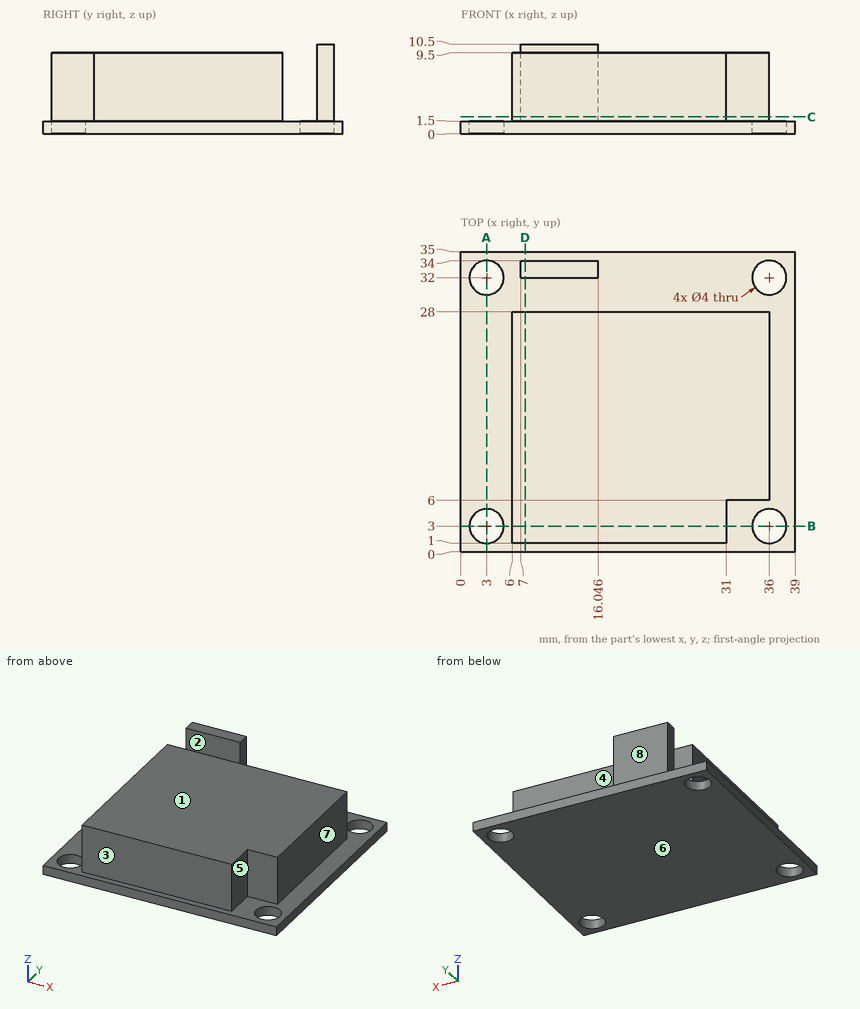
For this review, use the dimensioned drawing (mm, ordinates from the lowest corner) and the shaded views. A direction names the side the tool comes from. Coordinates: 2 decimals unless noted, no trailing zeros. Write each loop counter-clockwise with the first axis right and the second up, starting at its lowest first coordinate (ties: lowest second). Pieces come first, ordered by that corner, then holes. Notation, with made-up numbers: (-15, -19) - (33, -19) arc R15 ccw to (33, 5) - close; hole circle Ø4 at (-23.5, 36.5). An arc over 180 degrees is marked (long way). One line per item, written item: value.
1) Add section D-D (x = 7.5). State the section outline as (y, z) points, plus the area to 4 significant figures.
Answer sheet:
outline: (0, 0) - (35, 0) - (35, 1.5) - (34, 1.5) - (34, 10.5) - (32, 10.5) - (32, 1.5) - (28, 1.5) - (28, 9.5) - (1, 9.5) - (1, 1.5) - (0, 1.5) - close
area: 286.5 mm2
2) For the marked faces 5, 6, 7 and 8, list the 3-axis set-ups (+Z, -Z, +X, -X, +Y, -Y) from which the entire face can be reached by the end or side of a thin tool; tool diameter is ignored.
Answer sheet:
face 5: +Z, +X, -Y
face 6: -Z, +X, -X, +Y, -Y
face 7: +Z, +X, +Y, -Y
face 8: +Z, +X, -X, +Y
3) Insertion check: pin 1 (2 mm diameter, centred on x = 21.5, z = 6.5, fed in from +Y); pin 2 (2.5 mm diameter, centred on x = 13.5, z = 6.5, fed in from +Y); pin 3 (17.5 mm diameter, centred on x = 15, y = 15, fed in from +Z); pin 4 (3.5 mm diameter, centred on x = 3, y = 32, fed in from +Z). Each pin has a flat end and moves straight along its axis. Give the tip position at first contact, or say it passes through.
Answer sheet:
pin 1: stops at y = 28
pin 2: stops at y = 34
pin 3: stops at z = 9.5
pin 4: passes through
4) Add section A-A (x = 3). State the section outline as (y, z) points.
Answer sheet:
outline: (0, 0) - (1, 0) - (1, 1.5) - (0, 1.5) - close; (5, 0) - (30, 0) - (30, 1.5) - (5, 1.5) - close; (34, 0) - (35, 0) - (35, 1.5) - (34, 1.5) - close
5) Add section C-C (z = 2). State the section outline as (x, y) points, plus the area to 3 significant figures.
Answer sheet:
outline: (6, 1) - (31, 1) - (31, 6) - (36, 6) - (36, 28) - (6, 28) - close; (7, 32) - (16.05, 32) - (16.05, 34) - (7, 34) - close
area: 803 mm2
6) Add section B-B (y = 3). State the section outline as (x, z) points, plus the area to 4 significant figures.
Answer sheet:
outline: (0, 0) - (1, 0) - (1, 1.5) - (0, 1.5) - close; (5, 0) - (34, 0) - (34, 1.5) - (31, 1.5) - (31, 9.5) - (6, 9.5) - (6, 1.5) - (5, 1.5) - close; (38, 0) - (39, 0) - (39, 1.5) - (38, 1.5) - close
area: 246.5 mm2
7) To check wall thickness, follow probe 1 along Y at (x, z) = (36, 0.75); probe 2 along Y at (x, z) = (13, 5.25); probe 3 along Z at (x, y) = (6.5, 20.5). State the ranges of each line that lie inside material, in increasing order.
Answer sheet:
probe 1: y = 0 to 1, 5 to 30, 34 to 35
probe 2: y = 1 to 28, 32 to 34
probe 3: z = 0 to 9.5
8) Mouldability with a two-part tool opening along Y and no side actions: class the marked faces 1, 2, 3 and 4 as +Y half, -Y half, draft (parallel to the pull), parting line (faces both ways), or undercut.
Answer sheet:
face 1: draft
face 2: undercut
face 3: -Y half
face 4: undercut
